Geometry check sheet. Reference: drawing and pictorial views, mm from the part's lowest x, y, z. A direction names the side the tool comes from. Give positions to 0.01 mm unless a question says otherwise; leave off trailing zeros. Write each loop counter-clockwise with the first axis right and the second up, starting at its lowest first coordinate (ties: lowest second). Pieces come first, ordered by that corner, then holes. Notation, with made-up numbers: (28, -1.75) -> (41, -1.75) arc R26 ccw to (41, 16.25) -> close; hole circle Ø4 at (43, 39.25). An arc over 180 degrees is marked (long way). Use a Markdown table: item, result. Add a question column.
1. Gauge pin test, flat ends, axial feed: P1, Ø15, axis at x = 35, y = 26.5, coming from the -Z side; P2, Ø4, axis at x = 48, z = 21, coming from the +Y side; P3, Ø2, axis at x = 27.5, z = 27, coming from the +Y side; P4, Ø6, axis at y = 83.5, z = 10, coming from the -X side. Record the tip position at first contact, or that the pin passes through.
2. Cross-section at A-A (x = 38.5). Count the separate pieces of the cut face and the enclosed holes in it, then the cut area to 3 significant figures.
3. Scan lines: probe 1 along X at (y, z) = (89, 74); probe 2 along Z at (x, y) = (12.5, 57.5); probe 3 along Y at (x, z) = (38.5, 71.5). Record each from-to range of solid material in increasing order. Write a range as [from, to].
4. Release check for a two-part mould opening along X. For the marked faces 1, 2 and 3 record: released by +X, released by -X, zero draft, split by the parting line, or undercut.
5. Cross-section at C-C (y = 128). Enter the section's corners in (x, z) (1 decimal), then the cut area to 3 significant figures.
6. Cross-section at D-D (x = 55). Enter the section's corners in (y, z).
7. Set-up check for the marked faces 4, 5 and 6: record each of +Z, -Z, +X, -X, +Y, -Y from which the full face is reachable in a straight line by a thin tool's end or side.
8. Cross-section at B-B (z = 39.5). Enter the section's corners in (x, y).
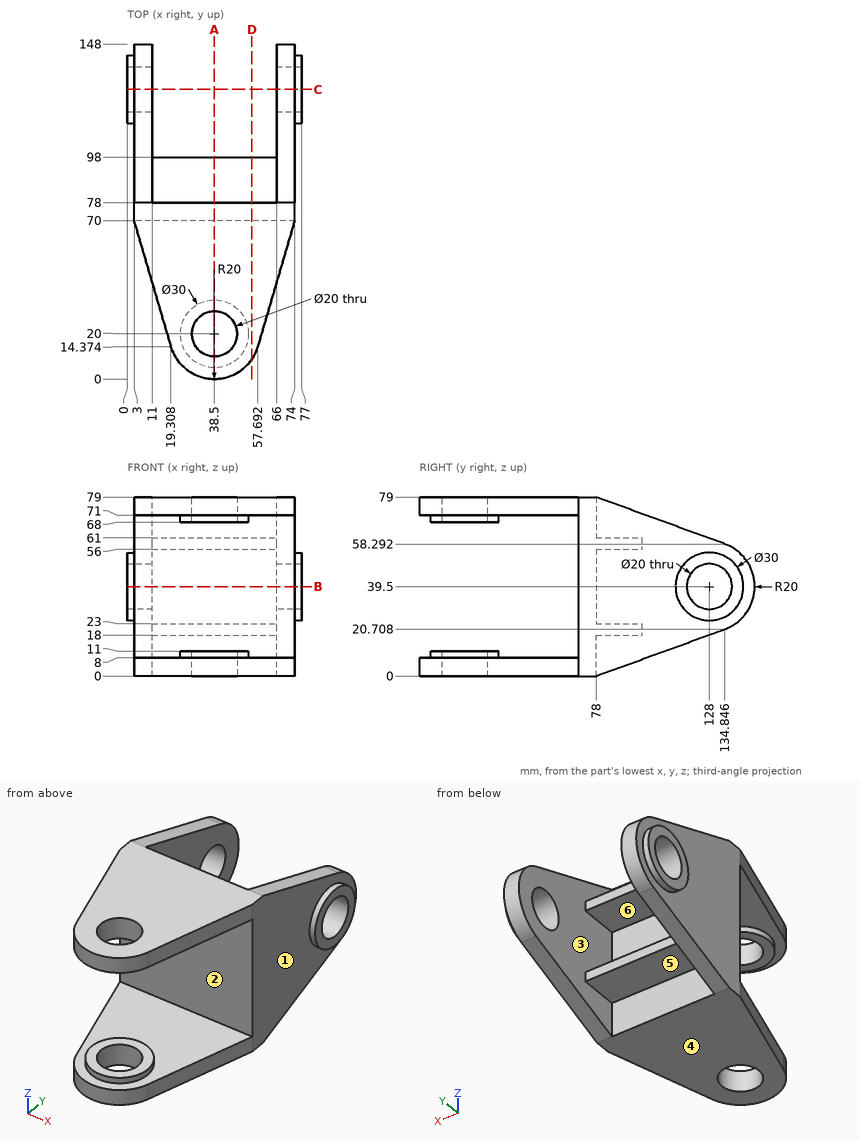
Worked answers:
| question | item | result |
|---|---|---|
| 1 | P1 | stops at z = 0 |
| 1 | P2 | stops at y = 98 |
| 1 | P3 | stops at y = 78 |
| 1 | P4 | stops at x = 3 |
| 2 | separate pieces | 3 |
| 2 | enclosed holes | 0 |
| 2 | area | 1,690 mm² |
| 3 | probe 1 | x = [3, 11], [66, 74] |
| 3 | probe 2 | z = [0, 8], [71, 79] |
| 3 | probe 3 | y = [0, 10], [30, 78] |
| 4 | face 1 | released by +X |
| 4 | face 2 | zero draft |
| 4 | face 3 | undercut |
| 5 | outline | (0, 24.5) -> (3, 24.5) -> (3, 18.2) -> (11, 18.2) -> (11, 29.5) -> (0, 29.5) -> close; (0, 49.5) -> (11, 49.5) -> (11, 60.8) -> (3, 60.8) -> (3, 54.5) -> (0, 54.5) -> close; (66, 18.2) -> (74, 18.2) -> (74, 24.5) -> (77, 24.5) -> (77, 29.5) -> (66, 29.5) -> close; (66, 49.5) -> (77, 49.5) -> (77, 54.5) -> (74, 54.5) -> (74, 60.8) -> (66, 60.8) -> close |
| 5 | area | 421 mm² |
| 6 | outline | (8.7, 0) -> (78, 0) -> (78, 18) -> (98, 18) -> (98, 23) -> (78, 23) -> (78, 56) -> (98, 56) -> (98, 61) -> (78, 61) -> (78, 79) -> (8.7, 79) -> (8.7, 71) -> (70, 71) -> (70, 8) -> (8.7, 8) -> close |
| 7 | face 4 | -Z, +X, -X, +Y, -Y |
| 7 | face 5 | -Z, +Y |
| 7 | face 6 | +Y |
| 8 | outline | (0, 113) -> (3, 113) -> (3, 70) -> (74, 70) -> (74, 113) -> (77, 113) -> (77, 118) -> (66, 118) -> (66, 78) -> (11, 78) -> (11, 118) -> (0, 118) -> close; (0, 138) -> (11, 138) -> (11, 148) -> (3, 148) -> (3, 143) -> (0, 143) -> close; (66, 138) -> (77, 138) -> (77, 143) -> (74, 143) -> (74, 148) -> (66, 148) -> close |
